Part model, mm, in its own coordinate system. Face numbers are marked on the shaded views. Coordinates: 2 decimals unless noted, no trailing zeros. Order: outer loops, then holes, each group sorted by start corner. A loop starts at its lowest first (then second) coordinate and runs counter-clockwise, first axis right, second up.
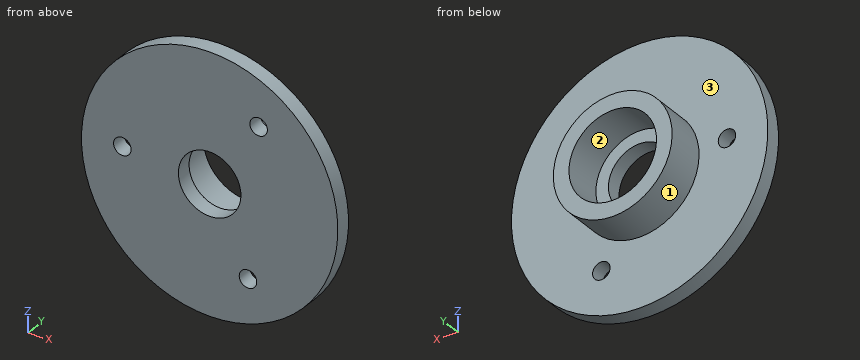
from build123d import *

# Parameters (mm, degrees)
ESQUISSE1_W      = 15.5
ESQUISSE1_H      = 2.5
ESQUISSE1_W_2    = 2.5
ESQUISSE1_H_2    = 6.3
ESQUISSE2_R      = 1.4
EXTRUSION1_DEPTH = 10


with BuildPart() as part:
    # Esquisse1 → Révolution1 (revolve)
    with BuildSketch(Plane.XY, mode=Mode.PRIVATE) as r_volution1_sk:
        with Locations((12.75, 1.25)):
            Rectangle(ESQUISSE1_W, ESQUISSE1_H)
        with Locations((8.25, 5.65)):
            Rectangle(ESQUISSE1_W_2, ESQUISSE1_H_2)
    revolve(r_volution1_sk.sketch.rotate(Axis((0, 0, 0), (0, 1, 0)), 90), axis=Axis((0, 0, 0), (0, 1, 0)))

    # Esquisse2 → Extrusion1 (cut)
    with BuildSketch(Plane.XZ):
        with Locations(Location((-13.965223749, 0.986167141, 0), (0, 0, 270))):
            Circle(ESQUISSE2_R)
        with Locations(Location((7.836657671, 11.601154966, 0), (0, 0, 270))):
            Circle(ESQUISSE2_R)
        with Locations(Location((6.128566078, -12.587322107, 0), (0, 0, 270))):
            Circle(ESQUISSE2_R)
    extrude(amount=-EXTRUSION1_DEPTH, mode=Mode.SUBTRACT)


solid = part.part
Q1. Mould opens along X. For the marked faces 1, 2 and 3 say: pulls with the +X half, pulls with the -X half, needs draft (parallel to the pull), parting line crosses it, or undercut.
Results list:
face 1: parting line crosses it
face 2: undercut
face 3: needs draft
Q2. Pin check, flat tips, straight feed: pin 1 Ø9 at (x, z) = (0, 0) entering from +Y; pin 2 Ø2 at (y, z) = (2, -4) entering from -X; pin 3 Ø3.5 at (x, z) = (-13.97, 0.99) entering from +Y. Stop position of each tip, or through.
Results list:
pin 1: passes through
pin 2: stops at x = -20.28
pin 3: stops at y = 2.5
Q3. Cut at A-A on x = 0. Write the cut outline in (y, z), and give its area (3 significant figures).
Results list:
outline: (0, -20.5) - (2.5, -20.5) - (2.5, -9.5) - (8.8, -9.5) - (8.8, -7) - (2.5, -7) - (2.5, -5) - (0, -5) - close; (0, 5) - (2.5, 5) - (2.5, 7) - (8.8, 7) - (8.8, 9.5) - (2.5, 9.5) - (2.5, 20.5) - (0, 20.5) - close
area: 109 mm2
Q4. Cut at D-D on z = 5.5. Write the cut outline in (x, y).
Results list:
outline: (-19.75, 0) - (19.75, 0) - (19.75, 2.5) - (7.75, 2.5) - (7.75, 8.8) - (4.33, 8.8) - (4.33, 2.5) - (-4.33, 2.5) - (-4.33, 8.8) - (-7.75, 8.8) - (-7.75, 2.5) - (-19.75, 2.5) - close
Q5. Cut at B-B on z = -13. Write the cut outline in (x, y), and give its area (3 significant figures).
Results list:
outline: (-15.85, 0) - (4.79, 0) - (4.79, 2.5) - (-15.85, 2.5) - close; (7.47, 0) - (15.85, 0) - (15.85, 2.5) - (7.47, 2.5) - close
area: 72.6 mm2
Q6. Cut at C-C on y = 4.75. Write the cut outline in (x, z), and give its area (3 significant figures).
Results list:
outline: circle Ø19 at (0, 0); hole circle Ø14 at (0, 0)
area: 130 mm2
Q7. Wall check: line 1 along X through (y, z) = (0.95, 0); line 2 along X through (y, z) = (6.25, 0); line 3 along Y through (x, z) = (14.5, 5). Give the ranges that are in metal, low to high.
Results list:
line 1: x = -20.5 to -14.96, -12.97 to -5, 5 to 20.5
line 2: x = -9.5 to -7, 7 to 9.5
line 3: y = 0 to 2.5
